Check sheet for the modelled part. Datum: model origin and axes. Units: mm. A direction names the side the tool comes from. Coordinates: 2 decimals unless noted, no trailing zeros. Write each loop counter-clockwise with the first axis right and the second up, starting at its lowest first coordinate (ties: lowest second). Pieces come first, ordered by that corner, then holes. Notation, with made-up numbers: (3, -20.5) -> (25, -20.5) arc R28 ccw to (25, 18.5) -> close; hole circle Ø4 at (63.5, -22.5). An arc over 180 degrees is marked (long way). Put each result on its own line as item: value.
```python
from build123d import *

# Parameters (mm, degrees)
SKETCH2_R           = 63.582050125
BOSS_EXTRUDE1_DEPTH = 2.54
DOME1_FACE_RADIUS   = 63.582050125
DOME1_HEIGHT        = 16.51
SKETCH3_R           = 63.582050125
SKETCH3_R_2         = 57.232050125
BOSS_EXTRUDE2_DEPTH = 50.8
SKETCH4_R           = 57.232050125
SKETCH4_R_2         = 50.882050125
BOSS_EXTRUDE3_DEPTH = 558.8
SKETCH5_R           = 50.882050125
BOSS_EXTRUDE4_DEPTH = 558.8


# Read off the part's stored shape, not the designer's step: Shell1
with BuildPart() as part:
    # Sketch2 → Boss-Extrude1 (new body)
    with BuildSketch(Plane.XY.offset(38.1)):
        with Locations((672.464575935, -1215.750984812)):
            Circle(SKETCH2_R)
    extrude(amount=BOSS_EXTRUDE1_DEPTH)

    # Dome1: a dome of height H over a round flat face of radius A is a cap of a sphere of radius (A * A + H * H) / (2 * H)
    dome1_r = (DOME1_FACE_RADIUS * DOME1_FACE_RADIUS + DOME1_HEIGHT * DOME1_HEIGHT) / (2 * DOME1_HEIGHT)
    dome1_base = Plane((672.464575935, -1215.750984812, 38.1), z_dir=(0, 0, -1))
    with Locations(dome1_base.offset(DOME1_HEIGHT - dome1_r)):
        dome1_ball = Sphere(dome1_r, mode=Mode.PRIVATE)
    add(split(dome1_ball, bisect_by=dome1_base, keep=Keep.TOP, mode=Mode.PRIVATE))

    # Sketch3 → Boss-Extrude2 (add)
    with BuildSketch(Plane.XY.offset(40.64)):
        with Locations((672.464575935, -1215.750984812)):
            Circle(SKETCH3_R)
        with Locations((672.464575935, -1215.750984812)):
            Circle(SKETCH3_R_2, mode=Mode.SUBTRACT)
    extrude(amount=BOSS_EXTRUDE2_DEPTH)

    # Sketch4 → Boss-Extrude3 (add)
    with BuildSketch(Plane.XY.offset(40.64)):
        with Locations((672.464575935, -1215.750984812)):
            Circle(SKETCH4_R)
        with Locations((672.464575935, -1215.750984812)):
            Circle(SKETCH4_R_2, mode=Mode.SUBTRACT)
    extrude(amount=BOSS_EXTRUDE3_DEPTH)

    # Sketch5 → Boss-Extrude4 (add)
    with BuildSketch(Plane.XY.offset(40.64)):
        with Locations((672.464575935, -1215.750984812)):
            Circle(SKETCH5_R)
    extrude(amount=BOSS_EXTRUDE4_DEPTH)

    # Shell1 outline → Shell1 (revolve, cut)
    with BuildSketch(Plane(origin=(672.464575935, -1215.750984812, 0), x_dir=(1, 0, 0), z_dir=(0, -1, 0))):
        with BuildLine():
            Line((57.232050162, 41.895123211), (57.232050125, 85.09))
            Line((57.232050125, 85.09), (50.882050125, 85.09))
            Line((50.882050125, 85.09), (50.882050125, 599.44))
            Line((50.882050125, 599.44), (0, 599.44))
            Line((0, 599.44), (0, 27.94))
            ThreePointArc((0, 27.94), (29.454426788, 31.47915065), (57.232050162, 41.895123211))
        make_face()
    revolve(axis=Axis((672.464575935, -1215.750984812, 0), (0, 0, 1)), mode=Mode.SUBTRACT)


solid = part.part
```
Q1. Cross-section at B-B (y = -1197.5). Record the cut outline in (x, z), plus the area to 3 significant figures.
Recorded:
outline: (611.56, 38.1) arc R129.41 ccw to (733.37, 38.1) -> (733.37, 91.44) -> (726.71, 91.44) -> (726.71, 599.44) -> (719.96, 599.44) -> (719.96, 85.09) -> (726.71, 85.09) -> (726.71, 41.9) arc R122.99 cw to (618.22, 41.9) -> (618.22, 85.09) -> (624.97, 85.09) -> (624.97, 599.44) -> (618.22, 599.44) -> (618.22, 91.44) -> (611.56, 91.44) -> close
area: 8,390 mm2
Q2. Cross-section at D-D (z = 515.5). Record the cut outline in (x, y), plus the area to 3 significant figures.
Recorded:
outline: circle Ø114.46 at (672.46, -1215.75); hole circle Ø101.76 at (672.46, -1215.75)
area: 2,160 mm2
Q3. Material ranges on line 1 along Y through (x, z) = (674, 257.5); line 2 along X through (y, z) = (-1172, 300); line 3 along X through (y, z) = (-1262, 500), recorded low to high.
Recorded:
line 1: y = -1272.96 to -1266.61, -1164.89 to -1158.54
line 2: x = 635.57 to 646.49, 698.44 to 709.36
line 3: x = 638.75 to 651.25, 693.68 to 706.18
Q4. Mould release check, pull along Z, two halves, no side actions. Record for faces 1 (the flat face through (634, -1249.4, 599.44)), 2 (the cylindrical face through (664.19, -1152.71, 64.4)), 3 (the cylindrical face through (665.014, -1159.006, 63.795)): released by +Z, released by -Z, zero draft, split by the parting line, or undercut.
Recorded:
face 1: released by +Z
face 2: zero draft
face 3: undercut
Q5. Tool access check on faces 4 (the flat face through (620, -1192, 91.44)), 5 (the flat face through (634, -1249.4, 85.09)). Record the directions out of +Z, -Z, +X, -X, +Y, -Y that give a thin tool (end or side, any length) a straight path to the whole face; none if there is none.
Recorded:
face 4: +Z
face 5: none
Q6. Cross-section at A-A (x = 640). Record the cut outline in (y, z).
Recorded:
outline: (-1270.42, 38.1) arc R126.59 ccw to (-1161.08, 38.1) -> (-1161.08, 91.44) -> (-1168.62, 91.44) -> (-1168.62, 599.44) -> (-1176.57, 599.44) -> (-1176.57, 85.09) -> (-1168.62, 85.09) -> (-1168.62, 41.9) arc R120.02 cw to (-1262.88, 41.9) -> (-1262.88, 85.09) -> (-1254.93, 85.09) -> (-1254.93, 599.44) -> (-1262.88, 599.44) -> (-1262.88, 91.44) -> (-1270.42, 91.44) -> close
Q7. Depth check by flat-ended pin: P1, Ø5, axis at x = 712.5, z = 458, coming from the -Y side; P2, Ø12, axis at y = -1166.5, z = 276, coming from the +X side; P3, Ø5, axis at x = 694, y = -1246.5, coming from the -Z side. Enter the tip coordinate at first touch or a pass-through.
Recorded:
P1: stops at y = -1258.96
P2: stops at x = 709.95
P3: stops at z = 26.38
Q8. Cross-section at C-C (z = 76). Record the cut outline in (x, y), plus the area to 3 significant figures.
Recorded:
outline: circle Ø127.16 at (672.46, -1215.75); hole circle Ø114.46 at (672.46, -1215.75)
area: 2,410 mm2
